For this review, take the finished solid that the model builds, in its own axes (mm). Give positions to 0.01 mm unless a question says otherwise; leave off trailing zeros. Loops run counter-clockwise (first coordinate to the right, second up) from the corner with the lowest first, then second, coordinate; pieces in that order, holes last. Notation, with made-up numbers: (12.5, -9.5) - (39.5, -9.5) arc R30 cw to (39.5, 21.5) - close; hole circle Ø11 at (57.25, 35.25). An arc over 180 degrees is marked (long way). Answer in a Markdown table with one row per item.
```python
from build123d import *

# Parameters (mm, degrees)
SKETCH1_R           = 5
BOSS_EXTRUDE1_DEPTH = 285
SKETCH2_R           = 4
BOSS_EXTRUDE2_DEPTH = 7
SKETCH3_R           = 3.175
BOSS_EXTRUDE3_DEPTH = 12
BOSS_EXTRUDE4_START = 6
SKETCH4_R           = 4
BOSS_EXTRUDE4_DEPTH = 6
CHAMFER1_SIZE       = 0.25


with BuildPart() as part:
    # Sketch1 → Boss-Extrude1 (new body)
    with BuildSketch(Plane.XY.offset(304)):
        with Locations(Location((0, 0, 0), (0, 0, 180))):
            Circle(SKETCH1_R)
    extrude(amount=-BOSS_EXTRUDE1_DEPTH)

    # Sketch2 → Boss-Extrude2 (add)
    with BuildSketch(Plane(origin=(0, 0, 19), x_dir=(-1, 0, 0), z_dir=(0, 0, -1))):
        with Locations(Location((0, 0, 0), (0, 0, 180))):
            Circle(SKETCH2_R)
    extrude(amount=BOSS_EXTRUDE2_DEPTH)

    # Sketch3 → Boss-Extrude3 (add)
    with BuildSketch(Plane(origin=(0, 0, 12), x_dir=(-1, 0, 0), z_dir=(0, 0, -1))):
        Circle(SKETCH3_R)
    extrude(amount=BOSS_EXTRUDE3_DEPTH)

    # Sketch4 → Boss-Extrude4 (add)
    with BuildSketch(Plane.XY.offset(304).offset(BOSS_EXTRUDE4_START)):
        Circle(SKETCH4_R)
    extrude(amount=-BOSS_EXTRUDE4_DEPTH)

    # Chamfer1
    chamfer1_edges = [part.edges().sort_by_distance(p)[0] for p in [
        (3.175, 0, 0),
        (-4, 0, 310),
        (5, 0, 304),
        (5, 0, 19),
        (-4, 0, 12),
    ]]
    chamfer(chamfer1_edges, length=CHAMFER1_SIZE)


solid = part.part
```
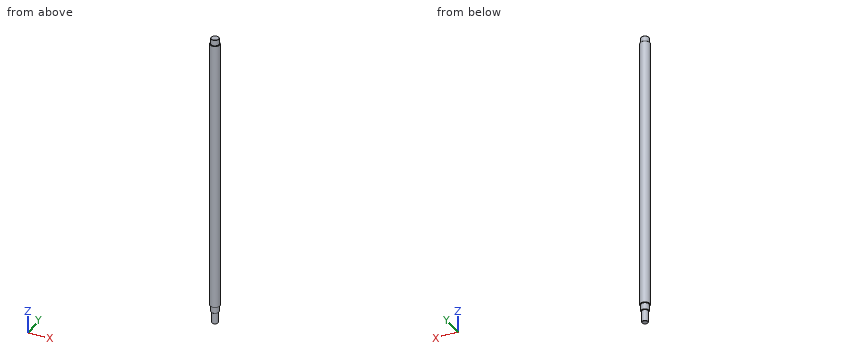
1. Wall thickness on line 1 (X direction, y = -3.25, z = 178); line 2 (Y direction, x = -0.5, z = 294.5); line 3 (Z direction, x = -1.5, y = 3.75): over which ranges is each line inside the solid? List them lowest first. Write a range as [from, to].
Values:
| item | result |
|---|---|
| line 1 | x = [-3.8, 3.8] |
| line 2 | y = [-4.97, 4.97] |
| line 3 | z = [19, 304] |
2. We need section A-A, the plane y = 0. Give the boundary of the cut face in (x, z) (3 decimals), and give its area (3 significant figures).
Values:
| item | result |
|---|---|
| outline | (-5, 19.25) - (-4.75, 19) - (-4, 19) - (-4, 12.25) - (-3.75, 12) - (-3.175, 12) - (-3.175, 0.25) - (-2.925, 0) - (2.925, 0) - (3.175, 0.25) - (3.175, 12) - (3.75, 12) - (4, 12.25) - (4, 19) - (4.75, 19) - (5, 19.25) - (5, 303.75) - (4.75, 304) - (4, 304) - (4, 309.75) - (3.75, 310) - (-3.75, 310) - (-4, 309.75) - (-4, 304) - (-4.75, 304) - (-5, 303.75) - close |
| area | 3,030 mm^2 |
3. We need section C-C, the plane z = 189. Give the boundary of the cut face in (x, y), and give its area (3 significant figures).
Values:
| item | result |
|---|---|
| outline | circle Ø10 at (0, 0) |
| area | 78.5 mm^2 |
4. Clearance check with flat-ended pins moving along their axes: pin 1 (1 mm diameter, centred on x = 4, y = -3.5, fed in from +Z); pin 2 (2 mm diameter, centred on y = 1.5, z = 179, fed in from +X); pin 3 (1 mm diameter, centred on x = 3.5, z = 147, fed in from +Y). State where each tip first meets the part, or that it passes through.
Values:
| item | result |
|---|---|
| pin 1 | stops at z = 303.93 |
| pin 2 | stops at x = 4.97 |
| pin 3 | stops at y = 4 |
